from build123d import *

# Parameters (mm, degrees)
SKETCH1_R           = 9.5
BOSS_EXTRUDE1_DEPTH = 7
SKETCH2_R           = 6.25
BOSS_EXTRUDE2_DEPTH = 7.5
SKETCH3_R           = 9.5
BOSS_EXTRUDE3_DEPTH = 1.5
SKETCH4_R           = 4.25
CUT_EXTRUDE1_DEPTH  = 17


with BuildPart() as part:
    # Sketch1 → Boss-Extrude1 (new body)
    with BuildSketch(Plane(origin=(0, 0, 0), x_dir=(1, 0, 0), z_dir=(0, 1, 0))):
        Circle(SKETCH1_R)
    extrude(amount=BOSS_EXTRUDE1_DEPTH)

    # Sketch2 → Boss-Extrude2 (add)
    with BuildSketch(Plane(origin=(0, 7, 0), x_dir=(1, 0, 0), z_dir=(0, 1, 0))):
        Circle(SKETCH2_R)
    extrude(amount=BOSS_EXTRUDE2_DEPTH)

    # Sketch3 → Boss-Extrude3 (add)
    with BuildSketch(Plane(origin=(0, 14.5, 0), x_dir=(1, 0, 0), z_dir=(0, 1, 0))):
        Circle(SKETCH3_R)
    extrude(amount=BOSS_EXTRUDE3_DEPTH)

    # Sketch4 → Cut-Extrude1 (cut, through all)
    with BuildSketch(Plane(origin=(0, 16, 0), x_dir=(1, 0, 0), z_dir=(0, 1, 0))):
        Circle(SKETCH4_R)
    extrude(amount=-CUT_EXTRUDE1_DEPTH, mode=Mode.SUBTRACT)


solid = part.part
The listing builds one solid part. Answer for the finished solid, in the listing's coordinates (mm). A direction names the side the tool comes from. Give positions to 0.01 mm unless a question says otherwise; leave off trailing zeros. Order: outer loops, then holes, each group sorted by start corner. A loop starts at its lowest first (then second) coordinate and runs counter-clockwise, first axis right, second up. Notation, with made-up numbers: (74, 24.25) -> (101, 24.25) arc R19 cw to (101, 61.25) -> close; hole circle Ø1 at (68, 17.25). An arc over 180 degrees is marked (long way). Put each result on its own line as item: value.
Item 1: For a pull along Y with two mould halves and no side action, classify faces 3 (the face through (4, 0, 2)), 4 (the face through (2.285, 8.112, -3.584)), 5 (the face through (6.2, 7, 2)) as released by +Y, released by -Y, zero draft, split by the parting line, or undercut.
Established:
face 3: released by -Y
face 4: zero draft
face 5: undercut
Item 2: A cutting plane is placed at D-D on z = 5. Give the vertices of the cut face in (x, y), plus the area to 3 significant figures.
Established:
outline: (-8.08, 0) -> (8.08, 0) -> (8.08, 7) -> (3.75, 7) -> (3.75, 14.5) -> (8.08, 14.5) -> (8.08, 16) -> (-8.08, 16) -> (-8.08, 14.5) -> (-3.75, 14.5) -> (-3.75, 7) -> (-8.08, 7) -> close
area: 194 mm^2
Item 3: Given P1, Ø4, axis at y = 10, z = 0, coming from the -X side; P2, Ø4, axis at y = 13, z = -7.5, coming from the +X side; P3, Ø5, axis at y = 8, z = 4.5, coming from the +X side, each flat-ended and moving along its own axis, determine where each tip first touches the part or whether it passes through.
Established:
P1: stops at x = -6.25
P2: stops at x = 7.22
P3: stops at x = 9.24
Item 4: For faces 1 (the face through (6.2, 14.5, 2)), 2 (the face through (4, 16, 2)), determine the directions among +Z, -Z, +X, -X, +Y, -Y from which every point of the face is accessible in a straight line to the end or side of a thin tool.
Established:
face 1: none
face 2: +Z, -Z, +X, -X, +Y
Item 5: A cutting plane is placed at C-C on y = 6. Give the vertices of the cut face in (x, z).
Established:
outline: circle Ø19 at (0, 0); hole circle Ø8.5 at (0, 0)
Item 6: Straight lines are drawn through the part: line 1 (X direction, y = 12, z = 0); line 2 (Y direction, x = -6.5, z = -3.75). For each, find the intervals that lie inside material, in ascending order.
Established:
line 1: x = -6.25 to -4.25, 4.25 to 6.25
line 2: y = 0 to 7, 14.5 to 16
Item 7: A cutting plane is placed at B-B on z = 0. Give the vertices of the cut face in (x, y).
Established:
outline: (-9.5, 0) -> (-4.25, 0) -> (-4.25, 16) -> (-9.5, 16) -> (-9.5, 14.5) -> (-6.25, 14.5) -> (-6.25, 7) -> (-9.5, 7) -> close; (4.25, 0) -> (9.5, 0) -> (9.5, 7) -> (6.25, 7) -> (6.25, 14.5) -> (9.5, 14.5) -> (9.5, 16) -> (4.25, 16) -> close
Item 8: A cutting plane is placed at A-A on x = 0. Give the vertices of the cut face in (y, z).
Established:
outline: (0, -9.5) -> (7, -9.5) -> (7, -6.25) -> (14.5, -6.25) -> (14.5, -9.5) -> (16, -9.5) -> (16, -4.25) -> (0, -4.25) -> close; (0, 4.25) -> (16, 4.25) -> (16, 9.5) -> (14.5, 9.5) -> (14.5, 6.25) -> (7, 6.25) -> (7, 9.5) -> (0, 9.5) -> close
